Geometry check sheet. Reference: drawing and pictorial views, mm from the part's lowest x, y, z. A direction names the side the tool comes from. Give positions to 0.01 mm unless a question says otherwise; leave off trailing zeros. Loops run counter-clockwise (first coordinate to the right, second up) from the corner with the lowest first, then second, coordinate; pieces in that order, holes last. Notation, with made-up numbers: (79, -32) - (95, -32) arc R19 cw to (95, -2) - close; hole circle Ø10 at (82.5, 27.5). An arc over 180 degrees is marked (long way). One line per question, with ' | ' between items. Start each with the question number.
1. Tool access check on the marked faces 1 and 2. Record the directions out of +Z, -Z, +X, -X, +Y, -Y that give a thin tool (end or side, any length) a straight path to the whole face; none if there is none.
2. Section check D-D, the plane z = 21. Enter the section's corners in (x, y), then the cut area to 3 significant figures.
3. Section check C-C, the plane x = 0.65. Enter the section's corners in (y, z), then the cut area to 3 significant figures.
4. Depth check by flat-ended pin: pin 1 Ø1 at (x, z) = (4, 21) entering from -Y; pin 2 Ø1.5 at (x, y) = (5, 7.5) entering from +Z; pin 3 Ø1 at (x, z) = (4, 43) entering from +Y. Enter the tip coordinate at first touch or a pass-through.
5. Thickness scan on line 1 along Y through (x, z) = (2, 40); line 2 along Z through (x, y) = (0.8, 11.5); line 3 along Z through (x, y) = (3.15, 9.75). Record the ranges inside material, lowest first. Write a range as from..to.
6. Section check A-A, the plane x = 3.9. Enter the section's corners in (y, z).
7. Section check B-B, the plane y = 9.25. Enter the section's corners in (x, z).
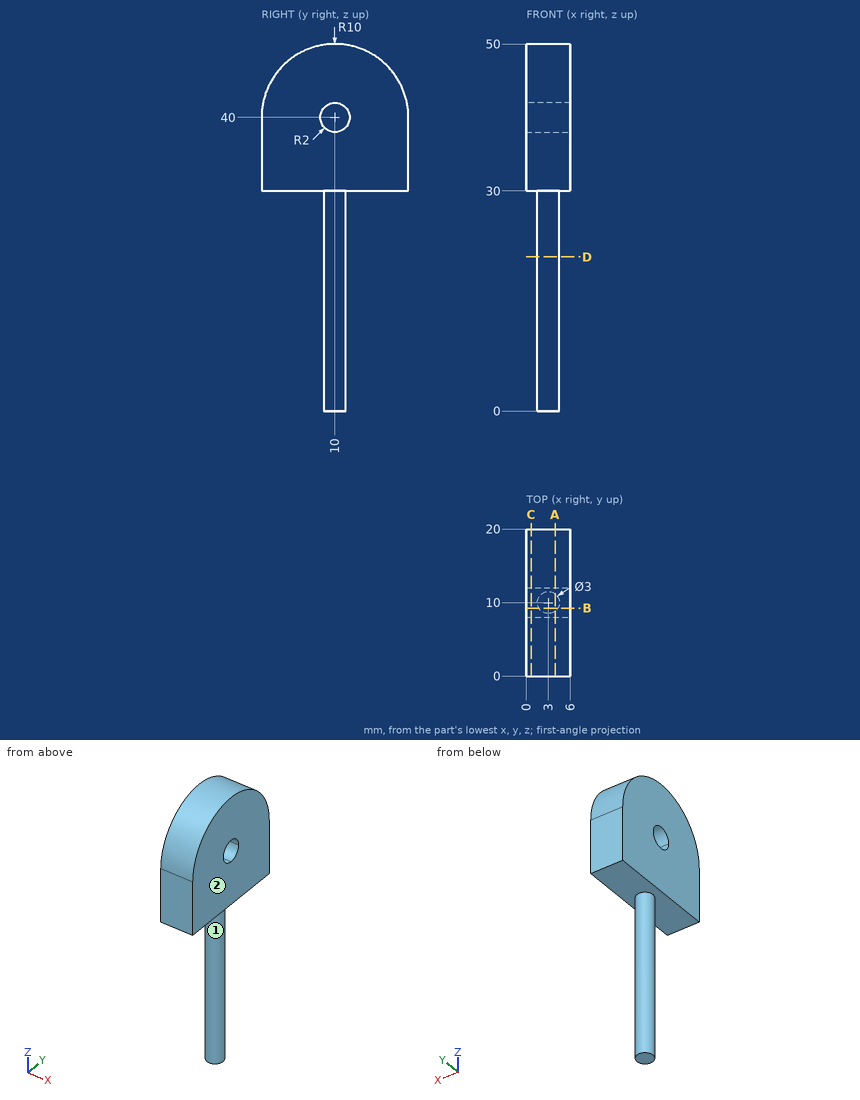
Results list:
1) face 1: -Z | face 2: +Z, -Z, +X, +Y, -Y
2) outline: circle Ø3 at (3, 10) | area: 7.07 mm²
3) outline: (0, 30) - (20, 30) - (20, 40) arc R10 ccw to (0, 40) - close; hole circle Ø4 at (10, 40) | area: 345 mm²
4) pin 1: y = 8.59 | pin 2: z = 49.85 | pin 3: y = 19.68
5) line 1: 0..8, 12..20 | line 2: 30..38.68, 41.32..49.89 | line 3: 0..38.02, 41.98..50
6) outline: (0, 30) - (8.8, 30) - (8.8, 0) - (11.2, 0) - (11.2, 30) - (20, 30) - (20, 40) arc R10 ccw to (0, 40) - close; hole circle Ø4 at (10, 40)
7) outline: (0, 30) - (1.7, 30) - (1.7, 0) - (4.3, 0) - (4.3, 30) - (6, 30) - (6, 38.15) - (0, 38.15) - close; (0, 41.85) - (6, 41.85) - (6, 49.97) - (0, 49.97) - close
